from build123d import *


with BuildPart() as part:
    # Front → Revolve1 (revolve)
    with BuildSketch(Plane.XY, mode=Mode.PRIVATE) as revolve1_sk:
        Polygon((0, 47.7), (4.04774101, 46.579378424), (8.49102763, 42.4), (8.49102763, 40.4), (5.258381655, 38.6), (5.258381655, 34.8), (7.058381655, 34.8), (7.058381655, 37.8), (8.558381655, 37.8), (9.619339829, 41.760349449), (7.760518893, 45.302211209), (5.258381655, 48.027887133), (3.61929083, 48.988814429), (2.757308273, 51.012915728), (0, 51.5), (-2.757308273, 51.012915728), (-3.61929083, 48.988814429), (-5.258381655, 48.027887133), (-7.760518893, 45.302211209), (-9.619339829, 41.760349449), (-8.558381655, 37.8), (-7.058381655, 37.8), (-7.058381655, 34.8), (-5.258381655, 34.8), (-5.258381655, 38.6), (-8.49102763, 40.4), (-8.49102763, 42.4), (-4.04774101, 46.579378424), align=None)
    revolve(revolve1_sk.sketch.rotate(Axis((0, 0, 0), (1, 0, 0)), 90), axis=Axis((0, 0, 0), (1, 0, 0)))


solid = part.part
Geometry check sheet. Reference: the model listing, model coordinates, mm. A direction names the side the tool comes from. Give positions to 0.01 mm unless a question says otherwise; leave off trailing zeros. Order: outer loops, then holes, each group sorted by start corner. A loop starts at its lowest first (then second) coordinate and runs counter-clockwise, first axis right, second up.
1) Material ranges on probe 1 along Y at (x, z) = (3, 12); probe 2 along Y at (x, z) = (-5.75, 16.5); probe 3 along Y at (x, z) = (7.55, 0), recorded low to high.
Results are:
probe 1: y = -48.99 to -45.31, 45.31 to 48.99
probe 2: y = -44.53 to -41.84, -35.2 to -30.64, 30.64 to 35.2, 41.84 to 44.53
probe 3: y = -45.53 to -43.29, -39.88 to -37.8, 37.8 to 39.88, 43.29 to 45.53
2) Tool access check on faces 1 (the cylindrical face through (-7.798, -11.354, 36.054)), 2 (the conical face through (-5.461, -11.628, 36.925)), 3 (the flat face through (7.058, 31, -17)), 4 (the cylindrical face through (6.171, 33.972, -7.544)). Record the directions out of +Z, -Z, +X, -X, +Y, -Y that give a thin tool (end or side, any length) a straight path to the whole face; none if there is none.
Results are:
face 1: -X
face 2: none
face 3: +X
face 4: +X, -X
3) Gauge pin test, flat ends, axial feed: pin 1 (5 mm diameter, centred on y = 28.5, z = -28.5, fed in from +X); pin 2 (4 mm diameter, centred on x = -6, y = 31.5, fed in from +Z); pin 3 (4 mm diameter, centred on x = 4, z = 2.5, fed in from +Y); pin 4 (5 mm diameter, centred on x = -3.5, z = 28, fed in from -Y). Record the tip position at first contact, or that the pin passes through.
Results are:
pin 1: stops at x = 9.62
pin 2: stops at z = 37.94
pin 3: stops at y = 51.1
pin 4: stops at y = -44.12
4) Cross-section at A-A (x = -1.25). Record the boundary of the cut face in (y, z).
Results are:
outline: circle Ø102.56 at (0, 0); hole circle Ø94.71 at (0, 0)
5) Draft check along Z on faces 5 (the flat face through (-8.491, 15.5, -37.5)), 6 (the flat face through (5.258, -34.5, -5.9)), 7 (the conical face through (9.503, -12.61, 40.043)). Enter one of: released by +Z, released by -Z, zero draft, split by the parting line, or undercut.
Results are:
face 5: undercut
face 6: undercut
face 7: split by the parting line
